```python
from build123d import *

# Parameters (mm, degrees)
SKETCH1_W           = 200
SKETCH1_H           = 150
BOSS_EXTRUDE1_DEPTH = 20
MIN_2_R             = 10.15
MIN_2_R_2           = 15.15
BOSS_EXTRUDE3_DEPTH = 30
MAX_LENTGH_R        = 10.15
MAX_LENTGH_R_2      = 15.15
BOSS_EXTRUDE4_DEPTH = 30
MAX_WIDTH_R         = 10.15
MAX_WIDTH_R_2       = 15.15
BOSS_EXTRUDE5_DEPTH = 30
MAX_2_R             = 10.15
MAX_2_R_2           = 15.15
BOSS_EXTRUDE6_DEPTH = 30


with BuildPart() as part:
    # Sketch1 → Boss-Extrude1 (new body)
    with BuildSketch(Plane.XY):
        Rectangle(SKETCH1_W, SKETCH1_H)
    extrude(amount=BOSS_EXTRUDE1_DEPTH)

    # min 2 → Boss-Extrude3 (add)
    with BuildSketch(Plane(origin=(0, 0, 0), x_dir=(-1, 0, 0), z_dir=(0, 0, -1))):
        with Locations((-50.3, -45.3)):
            Circle(MIN_2_R)
        with Locations((49.4, 44.4)):
            Circle(MIN_2_R_2)
    extrude(amount=BOSS_EXTRUDE3_DEPTH)

    # max - lentgh → Boss-Extrude4 (add)
    with BuildSketch(Plane(origin=(0, 0, 0), x_dir=(-1, 0, 0), z_dir=(0, 0, -1))):
        with Locations((-50, -44.7)):
            Circle(MAX_LENTGH_R)
        with Locations((50, 45.6)):
            Circle(MAX_LENTGH_R_2)
    extrude(amount=BOSS_EXTRUDE4_DEPTH)

    # max - width → Boss-Extrude5 (add)
    with BuildSketch(Plane(origin=(0, 0, 0), x_dir=(-1, 0, 0), z_dir=(0, 0, -1))):
        with Locations((-49.7, -45)):
            Circle(MAX_WIDTH_R)
        with Locations((50.6, 45)):
            Circle(MAX_WIDTH_R_2)
    extrude(amount=BOSS_EXTRUDE5_DEPTH)

    # max 2 → Boss-Extrude6 (add)
    with BuildSketch(Plane(origin=(0, 0, 0), x_dir=(-1, 0, 0), z_dir=(0, 0, -1))):
        with Locations((-49.7, -44.7)):
            Circle(MAX_2_R)
        with Locations((50.6, 45.6)):
            Circle(MAX_2_R_2)
    extrude(amount=BOSS_EXTRUDE6_DEPTH)


solid = part.part
```
Verification items for the finished model (mm, model axes). A direction names the side the tool comes from. Give positions to 0.01 mm unless a question says otherwise; leave off trailing zeros. Order: outer loops, then holes, each group sorted by start corner. A loop starts at its lowest first (then second) coordinate and runs counter-clockwise, first axis right, second up. Notation, with made-up numbers: (82.25, 64) - (122.25, 64) arc R25 cw to (122.25, 77) - close; hole circle Ø8 at (44.25, 79.5). An arc over 180 degrees is marked (long way). Answer as CSV lines item,"result". Start each with the question number.
Item 1: Section check D-D, the plane y = -66. Record the boundary of the cut face in (x, z), plus the area to 3 significant figures.
Item 2: Section check A-A, the plane z = -16.5. Record the boundary of the cut face in (x, y), plus the area to 3 significant figures.
Item 3: Access from +Z, -Z, +X, -X, +Y, -Y to the whole of each face (thin tool, end or side, straight path). Record for faces 1 (the face through (57.6, -52.35, -14.79)), 2 (the face through (100, -1, 10)).
Item 4: Material ranges on L1, parallel to Z at x = 53, y = 10; L2, parallel to X at y = 52, z = -4.5; L3, parallel to X at y = 47, z = -8.5, recorded low to high.
Item 5: Gauge pin test, flat ends, axial feed: pin 1 (10 mm diameter, centred on x = 35.5, z = -11, fed in from +Y); pin 2 (2 mm diameter, centred on x = -30, y = 3, fed in from -Z); pin 3 (1.5 mm diameter, centred on y = 37.5, z = -21, fed in from +X). Record the tip position at first contact, or that the pin passes through.
Item 6: Section check C-C, the plane y = -47.5. Record the boundary of the cut face in (x, z).
Item 7: Section check B-B, the plane x = -83.5. Record the boundary of the cut face in (y, z), plus the area to 3 significant figures.
Filled in:
1,outline,"(-100, 0) - (100, 0) - (100, 20) - (-100, 20) - close"
1,area,"4,000 mm^2"
2,outline,"(-65.75, 45.3) arc R15.15 ccw to (-56.77, 31.16) arc R15.15 ccw to (-36.16, 51.77) arc R15.15 ccw to (-50.3, 60.75) arc R15.15 ccw to start; (39.55, -44.85) arc R10.15 ccw to (45.46, -54.22) arc R10.15 ccw to (59.22, -40.46) arc R10.15 ccw to (49.85, -34.55) arc R10.15 ccw to start"
2,area,"1,120 mm^2"
3,face 1,"-Z"
3,face 2,"+Z, -Z, +X, +Y, -Y"
4,L1,"0 to 20"
4,L2,"-64.33 to -36.27"
4,L3,"-65.69 to -34.47"
5,pin 1,"y = -40.41"
5,pin 2,"z = 0"
5,pin 3,"x = -35.55"
6,outline,"(-100, 0) - (39.86, 0) - (39.86, -30) - (60.21, -30) - (60.21, 0) - (100, 0) - (100, 20) - (-100, 20) - close"
7,outline,"(-75, 0) - (75, 0) - (75, 20) - (-75, 20) - close"
7,area,"3,000 mm^2"
